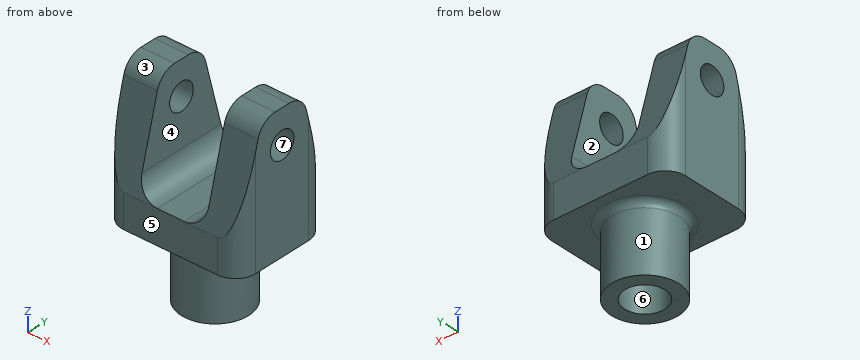
Autodesk Fusion 360 part; units mm, degrees
sketch "Sketch1" plane through (0, 0, 0) normal (0, 1, 0) x (1, 0, 0)
  line L0 (0, 0) -> (20, 0)
  line L1 (20, 0) -> (20, -20)
  line L2 (20, -20) -> (15, -20)
  line L3 (15, -20) -> (15, -5)
  line L4 (15, -5) -> (5, -5)
  line L5 (5, -5) -> (5, -20)
  line L6 (5, -20) -> (0, -20)
  line L7 (0, 0) -> (0, -20)
  dimension "d1" = 5
  dimension "d2" = 15
  dimension "d3" = 10
extrude "Extrude1" add sketch "Sketch1" along normal blind 15
sketch "Sketch2" plane through (20, 0, 0) normal (1, 0, 0) x (0, 1, 0)
  line L0 (0, 20) -> (0, 0)
  line L1 (0, 0) -> (15, 0)
  line L2 (15, 0) -> (15, 20)
  line L3 (15, 20) -> (0, 20)
  line L4 (7.5, 20) -> (7.5, 15)
  circle A0 centre (7.5, 15) radius 2
  dimension "d6" = 5
  dimension "d7" = 4
extrude "Extrude2" cut sketch "Sketch2" against normal through all contours A0
sketch "Sketch3" plane through (0, 0, 0) normal (0, 0, -1) x (1, 0, 0)
  line L0 (20, 0) -> (0, 0)
  line L1 (0, 0) -> (0, -15)
  line L2 (0, -15) -> (20, -15)
  line L3 (20, -15) -> (20, 0)
  line L4 (10, 0) -> (10, -7.5)
  circle A0 centre (10, -7.5) radius 5
  circle A1 centre (10, -7.5) radius 3
  dimension "d9" = 7.5
  dimension "d10" = 10
  dimension "d11" = 6
extrude "Extrude3" add sketch "Sketch3" along normal blind 10 contours A0
sketch "Sketch4" plane through (20, 0, 0) normal (1, 0, 0) x (0, 1, 0)
  circle A0 centre (7.5, 15) radius 2
  line L0 (0, 20) -> (0, 0)
  line L1 (0, 0) -> (15, 0)
  line L2 (15, 0) -> (15, 20)
  line L3 (15, 20) -> (0, 20)
  line L4 (0, 5) -> (4.0192, 20)
  line L5 (0, 5) -> (15, 5)
  line L6 (15, 5) -> (10.9808, 20)
  dimension "d14" = 75
  dimension "d15" = 75
extrude "Extrude4" cut sketch "Sketch4" against normal through all contours L0 L3 L4 | L2 L3 L6
fillet "Fillet1" radius 3 4 edges at (2.5, 4.0192, 20) (2.5, 10.9808, 20) (17.5, 4.0192, 20) (17.5, 10.9808, 20)
fillet "Fillet2" radius 3 6 edges at (0, 0, 2.5) (20, 0, 2.5) (20, 15, 2.5) (5, 7.5, 5) (15, 7.5, 5) (0, 15, 2.5)
fillet "Fillet3" radius 1 1 edges at (5.3384, 5.6919, 0)
Here's how the part is built. I have some questions about the finished solid (model axes, mm). Face numbers are marked on the shaded views. A direction names the side the tool comes from. Coordinates: 2 decimals unless noted, no trailing zeros. Write each loop counter-clockwise with the first axis right and the second up, starting at its lowest first coordinate (ties: lowest second). Pieces come first, ordered by that corner, then holes.
1) I'm going to push flat-ended pins straight in: pin 1 (6 mm diameter, centred on x = 2.5, y = 3, fed in from -Z); pin 2 (1.5 mm diameter, centred on x = 12.5, y = 3.5, fed in from +Z); pin 3 (2 mm diameter, centred on x = 16.5, y = 9, fed in from -Z). Where does each tip first touch, or does it pass through?
Filled in:
pin 1: stops at z = -0.03
pin 2: stops at z = 5.27
pin 3: stops at z = -0.06
2) Thinking about a two-plate mould opening in Y: for the marked faces 4, 5, 6 and 7, which applies, +Y half, -Y half, draft (parallel to the pull), parting line (faces both ways), or undercut?
Filled in:
face 4: draft
face 5: -Y half
face 6: undercut
face 7: undercut
3) If we section it at C-C (x = 10): List the corners of the cut face in (y, z) for me.
Filled in:
outline: (0, 0) - (1.5, 0) arc R1 cw to (2.5, -1) - (2.5, -10) - (4.5, -10) - (4.5, 0) - (10.5, 0) - (10.5, -10) - (12.5, -10) - (12.5, -1) arc R1 cw to (13.5, 0) - (15, 0) - (15, 5) - (0, 5) - close
4) If I drill on line 1 (X direction, y = 7.5, z = -5); line 2 (Y direction, x = 10, z = -5); line 3 (Z direction, x = 16.95, y = 7.5), over which ranges is the centre line in solid material (lowest first)?
Filled in:
line 1: x = 5 to 7, 13 to 15
line 2: y = 2.5 to 4.5, 10.5 to 12.5
line 3: z = 0 to 13, 17 to 20
5) Which directions (+Z, -Z, +X, -X, +Y, -Y) give clear straight access to the entire face, cutting with the end or side of a thin tool? Please do the marked faces 1, 2 and 3.
Filled in:
face 1: -Z
face 2: +Z, +Y, -Y
face 3: +Z, +X, -X, -Y
6) If we section it at B-B (z = 10.75): List the corners of the cut face in (x, y) for me.
Filled in:
outline: (0, 3) arc R3 ccw to (0.38, 1.54) - (5, 1.54) - (5, 13.46) - (0.38, 13.46) arc R3 ccw to (0, 12) - close; (15, 1.54) - (19.62, 1.54) arc R3 ccw to (20, 3) - (20, 12) arc R3 ccw to (19.62, 13.46) - (15, 13.46) - close
7) If we section it at D-D (x = 17.5): List the corners of the cut face in (y, z) for me.
Filled in:
outline: (0.04, 0) - (14.96, 0) - (14.96, 5.16) - (11.58, 17.78) arc R3 ccw to (8.68, 20) - (6.32, 20) arc R3 ccw to (3.42, 17.78) - (0.04, 5.16) - close; hole circle Ø4 at (7.5, 15)
8) If we section it at A-A (y = 7.5): List the corners of the cut face in (x, z) for me.
Filled in:
outline: (0, 0) - (4, 0) arc R1 cw to (5, -1) - (5, -10) - (7, -10) - (7, 0) - (13, 0) - (13, -10) - (15, -10) - (15, -1) arc R1 cw to (16, 0) - (20, 0) - (20, 13) - (15, 13) - (15, 8) arc R3 cw to (12, 5) - (8, 5) arc R3 cw to (5, 8) - (5, 13) - (0, 13) - close; (0, 17) - (5, 17) - (5, 20) - (0, 20) - close; (15, 17) - (20, 17) - (20, 20) - (15, 20) - close
